Build history of the part. All positions in model axes, mm. Give positions to 0.01 mm unless a question says otherwise; leave off trailing zeros. Write each loop counter-clockwise with the first axis right and the second up, starting at its lowest first coordinate (ties: lowest second). Pieces come first, ordered by that corner, then holes. Notation, with made-up numbers: M 14.5,47 L 18.5,47 A23 cw 18.5,55 Z; hole C 34,52.5 d6. An arc over 180 degrees is marked long. Return JSON: item names as keys, results as strings. Group by question number.
Q1. Band-saw the part on B-B, the plane z = -375. Give the cut face in (x, y).
Q2. Wall check: probe 1 along Z at (x, y) = (25, -7.5); probe 2 along Z at (x, y) = (21.5, -10.25); probe 3 along Z at (x, y) = (46.5, -9.5). Give the ranges that are in metal, low to high.
Q3. Band-saw the part on C-C, the plane z = -736. Give the cut face in (x, y), then the cut area to 3 significant figures.
Q4. Pull direction Z, two halves, no side cores. Call faces 1 (the flat face through (0, -6, -370)), 2 (the cylindrical face through (23.645, -5.916, -381.101)): +Z half, -Z half, draft (parallel to the pull), parting line (faces both ways), or undercut.
Q5. Flat gauge pins, fed straight in: pin 1 Ø14.5 at (x, z) = (25, -375) entering from -Y; pin 2 Ø9.5 at (x, z) = (25, -14) entering from +Y; pin 3 Ø5 at (x, y) = (12.5, -6.5) entering from +Z. Where does each tip first touch, or does it go through?
Q6. Band-saw the part on A-A, the plane y = -9.25. Give the cut face in (x, z), then the cut area to 3 significant figures.
from build123d import *

# Parameters (mm, degrees)
F0_R     = 6.25
F0_R_2   = 7.75
F1_DEPTH = 12


with BuildPart() as f1:
    # F0 (on Front) → F1 (new body)
    with BuildSketch(Plane.XZ):
        with BuildLine():
            Line((0, -25), (0, -725))
            Line((0, -725), (50, -725))
            Line((50, -725), (50, -25))
            ThreePointArc((50, -25), (42.67767, -7.32233), (25, 0))
            ThreePointArc((25, 0), (7.32233, -7.32233), (0, -25))
        make_face()
        with Locations((25, -375)):
            Circle(F0_R, mode=Mode.SUBTRACT)
        with Locations((25, -14)):
            Circle(F0_R_2, mode=Mode.SUBTRACT)
        with BuildLine():
            Line((50, -725), (0, -725))
            ThreePointArc((0, -725), (7.32233, -742.67767), (25, -750))
            ThreePointArc((25, -750), (42.67767, -742.67767), (50, -725))
        make_face()
        with Locations((25, -736)):
            Circle(F0_R_2, mode=Mode.SUBTRACT)
    extrude(amount=F1_DEPTH)


solid = f1.part
From the geometry:
{
 "1": {"outline": "M 0,-12 L 18.75,-12 L 18.75,0 L 0,0 Z; M 31.25,-12 L 50,-12 L 50,0 L 31.25,0 Z"},
 "2": {"probe 1": "z = -750 to -743.75, -728.25 to -381.25, -368.75 to -21.75, -6.25 to 0", "probe 2": "z = -749.75 to -742.91, -729.09 to -380.18, -369.82 to -20.91, -7.09 to -0.25", "probe 3": "z = -737.76 to -12.24"},
 "3": {"outline": "M 2.55,-12 L 17.25,-12 L 17.25,0 L 2.55,0 Z; M 32.75,-12 L 47.45,-12 L 47.45,0 L 32.75,0 Z", "area": "353 mm^2"},
 "4": {"face 1": "draft", "face 2": "undercut"},
 "5": {"pin 1": "stops at y = -12", "pin 2": "passes through", "pin 3": "stops at z = -2.09"},
 "6": {"outline": "M 0,-725 A25 ccw 25,-750 A25 ccw 50,-725 L 50,-25 A25 ccw 25,0 A25 ccw 0,-25 Z; hole C 25,-736 d15.5; hole C 25,-14 d15.5; hole C 25,-375 d12.5", "area": "36,500 mm^2"}
}
